```python
from build123d import *

# Parameters (mm, degrees)
BOSS_EXTRUDE1_DEPTH              = 10
F_8_0_8_DIAMETER_HOLE1_D         = 8
F_1_8_27_NPSM_TAPPED_HOLE1_D     = 9.0932
F_1_8_27_NPSM_TAPPED_HOLE1_DEPTH = 22.99
F_1_8_27_NPSM_TAPPED_HOLE1_TIP   = 2.73187289


with BuildPart() as part:
    # Sketch1 → Boss-Extrude1 (new body)
    with BuildSketch(Plane.XY):
        with BuildLine():
            Line((-10, -10), (-10, 80))
            ThreePointArc((-10, 80), (-7.071067812, 87.071067812), (0, 90))
            Line((0, 90), (210, 90))
            Line((210, 90), (210, 0))
            ThreePointArc((210, 0), (207.071067812, -7.071067812), (200, -10))
            Line((200, -10), (-10, -10))
        make_face()
        Polygon((42.360679775, 70), (190, 70), (190, 10.94427191), align=None, mode=Mode.SUBTRACT)
        Polygon((10, 10), (10, 69.05572809), (157.639320225, 10), align=None, mode=Mode.SUBTRACT)
    extrude(amount=BOSS_EXTRUDE1_DEPTH)

    # Ø8.0 (8) Diameter Hole1 (through all)
    with Locations(Plane(origin=(0, -10, 0), x_dir=(-1, 0, 0), z_dir=(0, -1, 0))):
        with Locations((5, -5)):
            Hole(F_8_0_8_DIAMETER_HOLE1_D / 2)

    # 1/8-27 NPSM Tapped Hole1
    with Locations(Plane(origin=(0, 90, 0), x_dir=(1, 0, 0), z_dir=(0, 1, 0))):
        with Locations((202.585893874, -5)):
            Hole(F_1_8_27_NPSM_TAPPED_HOLE1_D / 2, depth=F_1_8_27_NPSM_TAPPED_HOLE1_DEPTH)
            with Locations((0, 0, -(F_1_8_27_NPSM_TAPPED_HOLE1_DEPTH + F_1_8_27_NPSM_TAPPED_HOLE1_TIP / 2))):  # 118° drill point
                Cone(0, F_1_8_27_NPSM_TAPPED_HOLE1_D / 2, F_1_8_27_NPSM_TAPPED_HOLE1_TIP, mode=Mode.SUBTRACT)


solid = part.part
```
Here's how the part is built. I have some questions about the finished solid (model axes, mm). A direction names the side the tool comes from. Coordinates: 2 decimals unless noted, no trailing zeros. Loops run counter-clockwise (first coordinate to the right, second up) from the corner with the lowest first, then second, coordinate; pieces in that order, holes last. Notation, with made-up numbers: (33, -7.75) - (43, -7.75) arc R19 cw to (43, -1.75) - close; hole circle Ø1 at (48, -27). An arc over 180 degrees is marked (long way). Return JSON: item names as keys, results as strings. Group by question number.
Item 1: If we section it at A-A on y = 54: Write out the boundary of the cut face in (x, z).
Item 2: We'd pull the mould along Y, two halves only. Please class faces 3 (the face through (198.25, 78.34, 3.63)), 4 (the face through (82.79, 39.94, 4.93)), 5 (the face through (-9.109, 84.126, 3.819)), 6 (the face through (190, 41, 5)): +Y half, -Y half, draft (parallel to the pull), parting line (faces both ways), or undercut.
Item 3: I need wall thicknesses on line 1 (X direction, y = 10.5, z = 2.25); line 2 (Y direction, x = 92, z = 6.25); line 3 (Y direction, x = 63.5, z = 0.5). Which ranges of each line are inside material? Lowest first, please. Write a range as from..to.
Item 4: On a 3-axis mill with a long thin cutter (end or side, diameter ignored), from which of +Z, -Z, +X, -X, +Y, -Y can I reach the whole of each face in a straight line? I mean faces 1 (the face through (104, 90, 5)), 2 (the face through (10, 39, 5)). Say none if no direction works.
Item 5: If we section it at C-C on z = 3: State how many separate pieces and enclosed holes the cut face has, and give its area (3 significant figures).
Item 6: If we section it at B-B on x = 89.5: Write out the boundary of the cut face in (y, z), and give its area (3 significant figures).
Item 7: If we section it at D-D on y = 5: Write out the boundary of the cut face in (x, z).
Calculated:
{
 "1": {"outline": "(-10, 0) - (10, 0) - (10, 10) - (-10, 10) - close; (47.64, 0) - (82.36, 0) - (82.36, 10) - (47.64, 10) - close; (190, 0) - (210, 0) - (210, 10) - (190, 10) - close; hole circle Ø8 at (-5, 5)"},
 "2": {"face 3": "draft", "face 4": "undercut", "face 5": "+Y half", "face 6": "undercut"},
 "3": {"line 1": "x = -10..-7.9, -2.1..10, 156.39..210", "line 2": "y = -10..10, 36.26..50.14, 70..90", "line 3": "y = -10..10, 47.66..61.54, 70..90"},
 "4": {"face 1": "+Z, -Z, +X, -X, +Y", "face 2": "+Z, -Z"},
 "5": {"separate pieces": "2", "enclosed holes": "2", "area": "12,400 mm^2"},
 "6": {"outline": "(-10, 0) - (10, 0) - (10, 10) - (-10, 10) - close; (37.26, 0) - (51.14, 0) - (51.14, 10) - (37.26, 10) - close; (70, 0) - (90, 0) - (90, 10) - (70, 10) - close", "area": "539 mm^2"},
 "7": {"outline": "(-10, 0) - (210, 0) - (210, 10) - (-10, 10) - close; hole circle Ø8 at (-5, 5)"}
}
